Work out the finished part from the listing and answer in its coordinate system (mm). A direction names the side the tool comes from. Coordinates: 2 decimals unless noted, no trailing zeros. Order: outer loops, then holes, each group sorted by start corner. A loop starts at its lowest first (then second) coordinate and runs counter-clockwise, first axis right, second up. Notation, with made-up numbers: (21.25, 62.25) -> (58.25, 62.25) arc R10 ccw to (58.25, 75.25) -> close; hole circle Ø8 at (51, 85). An arc over 180 degrees is marked (long way). Use one line per item in the form item = value.
Autodesk Inventor part; units mm, degrees
ref_plane "type_gl_n_bm_XY" through (0, 0, 0) normal (1, 0, 0) x (0, -1, 0)
ref_plane "type_gl_n_bm_YZ" through (0, 0, 0) normal (0, -1, 0) x (0, 0, -1)
ref_plane "type_gl_n_bm_ZX" through (0, 0, 0) normal (0, 0, -1) x (1, 0, 0)
sketch "Sketch_1" plane through (0, 0, 0) normal (1, 0, 0) x (0, 1, 0)
  line L0 (27.33, 32.99) -> (-27.33, 32.99)
  line L1 (-27.33, 32.99) -> (-32.99, 27.33)
  line L2 (-32.99, 27.33) -> (-32.99, -27.33)
  line L3 (-32.99, -27.33) -> (-27.33, -32.99)
  line L4 (-27.33, -32.99) -> (27.33, -32.99)
  line L5 (27.33, -32.99) -> (32.99, -27.33)
  line L6 (32.99, -27.33) -> (32.99, 27.33)
  line L7 (32.99, 27.33) -> (27.33, 32.99)
extrude "Extrusion1" add sketch "Sketch_1" along normal blind 8
sketch "Sketch_2" plane through (0, 0, 0) normal (0, 0, 1) x (1, 0, 0)
  line L0 (40, 0) -> (8, 0)
  line L1 (8, 0) -> (8, 30)
  line L2 (8, 30) -> (40, 30)
  line L3 (40, 30) -> (40, 0)
  line L4 (40, 0) -> (8, 0)
revolve "Revolution1" add sketch "Sketch_2" angle 360 about axis through (40, 0, 0) along (1, 0, 0)
sketch "Sketch_3" plane through (40, 0, 0) normal (1, 0, 0) x (0, 0, -1)
  line L0 (-33, 27.34) -> (-33, -27.34)
  line L1 (-33, -27.34) -> (-27.34, -33)
  line L2 (-27.34, -33) -> (27.34, -33)
  line L3 (27.34, -33) -> (33, -27.34)
  line L4 (33, -27.34) -> (33, 27.34)
  line L5 (33, 27.34) -> (27.34, 33)
  line L6 (27.34, 33) -> (-27.34, 33)
  line L7 (-27.34, 33) -> (-33, 27.34)
extrude "Extrusion2" add sketch "Sketch_3" along normal blind 8
sketch "Sketch4" plane through (48, 0, 0) normal (1, 0, 0) x (0, 0, -1)
  point P0 (0, 0)
hole "Drilling 1" at (48, 0, 0) direction (-1, 0, 0) diameter 38.15 depth 8
sketch "Sketch5" plane through (40, 0, 0) normal (1, 0, 0) x (0, 0, -1)
  point P0 (0, 0)
hole "Drilling 2" at (40, 0, 0) direction (-1, 0, 0) diameter 50 depth 40
sketch "Sketch_7" plane through (0, 26.87, 0) normal (0, 1, 0) x (1, 0, 0)
  line L0 (13, 26.87) -> (8, 26.87)
  line L1 (8, 26.87) -> (8, 31.12)
  line L2 (8, 31.12) -> (13, 31.12)
  line L3 (13, 31.12) -> (13, 26.87)
  line L4 (13, 26.87) -> (8, 26.87)
revolve "Revolution2" add sketch "Sketch_7" angle 360 about axis through (13, 26.87, -26.87) along (1, 0, 0)
sketch "Sketch_8" plane through (0, 26.87, 0) normal (0, 1, 0) x (1, 0, 0)
  line L0 (13, -26.87) -> (8, -26.87)
  line L1 (8, -26.87) -> (8, -22.62)
  line L2 (8, -22.62) -> (13, -22.62)
  line L3 (13, -22.62) -> (13, -26.87)
  line L4 (13, -26.87) -> (8, -26.87)
revolve "Revolution3" add sketch "Sketch_8" angle 360 about axis through (13, 26.87, 26.87) along (1, 0, 0)
sketch "Sketch8" plane through (48, 0, 0) normal (1, 0, 0) x (0, 0, -1)
  point P0 (-23.57, 23.57)
hole "Drilling 3" at (48, 23.57, 23.57) direction (-1, 0, 0) diameter 3.242 depth 8 countersink diameter 4 countersink angle 90
sketch "Sketch9" plane through (48, 0, 0) normal (1, 0, 0) x (0, 0, -1)
  point P0 (-23.57, -23.57)
hole "Drilling 4" at (48, -23.57, 23.57) direction (-1, 0, 0) diameter 3.242 depth 8 countersink diameter 4 countersink angle 90
sketch "Sketch10" plane through (48, 0, 0) normal (1, 0, 0) x (0, 0, -1)
  point P0 (23.57, 23.57)
hole "Drilling 5" at (48, 23.57, -23.57) direction (-1, 0, 0) diameter 3.242 depth 8 countersink diameter 4 countersink angle 90
sketch "Sketch11" plane through (48, 0, 0) normal (1, 0, 0) x (0, 0, -1)
  point P0 (23.57, -23.57)
hole "Drilling 6" at (48, -23.57, -23.57) direction (-1, 0, 0) diameter 3.242 depth 8 countersink diameter 4 countersink angle 90
sketch "Sketch_9" plane through (0, -26.87, 0) normal (0, 1, 0) x (1, 0, 0)
  line L0 (13, 26.87) -> (8, 26.87)
  line L1 (8, 26.87) -> (8, 31.12)
  line L2 (8, 31.12) -> (13, 31.12)
  line L3 (13, 31.12) -> (13, 26.87)
  line L4 (13, 26.87) -> (8, 26.87)
revolve "Revolution4" add sketch "Sketch_9" angle 360 about axis through (13, -26.87, -26.87) along (1, 0, 0)
sketch "Sketch_10" plane through (0, -26.87, 0) normal (0, 1, 0) x (1, 0, 0)
  line L0 (13, -26.87) -> (8, -26.87)
  line L1 (8, -26.87) -> (8, -22.62)
  line L2 (8, -22.62) -> (13, -22.62)
  line L3 (13, -22.62) -> (13, -26.87)
  line L4 (13, -26.87) -> (8, -26.87)
revolve "Revolution5" add sketch "Sketch_10" angle 360 about axis through (13, -26.87, 26.87) along (1, 0, 0)
sketch "Sketch_33" plane through (0, 0, 0) normal (0, 1, 0) x (-1, 0, 0)
  line L0 (0, -17.5) -> (0, 17.5)
  line L1 (0, 17.5) -> (-33, 17.5)
  arc A0 (-33, 17.5) -> (-38, 12.5) centre (-33, 12.5) ccw
  line L2 (-38, 12.5) -> (-38, -12.5)
  arc A1 (-38, -12.5) -> (-33, -17.5) centre (-33, -12.5) ccw
  line L3 (-33, -17.5) -> (0, -17.5)
extrude "Extrusion3" cut sketch "Sketch_33" along normal blind 33
ref_plane "type_gl_n_bm_XY" through (0, 0, 0) normal (1, 0, 0) x (0, -1, 0)
ref_plane "type_gl_n_bm_YZ" through (0, 0, 0) normal (0, -1, 0) x (0, 0, -1)
ref_plane "type_gl_n_bm_ZX" through (0, 0, 0) normal (0, 0, -1) x (1, 0, 0)
properties part number "GL20NU1 Y Motor bracket"
(1) Each of these flat-tipped pins is pushed along its axis until it touches: P1, Ø3, axis at x = 26, y = -7.5, coming from the -Z side; P2, Ø5, axis at x = 21.5, y = 15.5, coming from the -Z side; P3, Ø8, axis at x = 26, z = -7.5, coming from the +Y side; P4, Ø3, axis at y = -9.5, z = 15, coming from the +X side. Where does it stop, or does it pass through?
Data:
P1 = -29.39
P2 = -27.04
P3 = -22.2
P4 = 48
(2) Straight lines are drawn through the part: line 1 along Z through (x, y) = (43.25, -23.57); line 2 along Y through (x, z) = (42, -23). For each, find the intervals that lie inside material, in ascending order.
Data:
line_1 = -33 to -25.19, -21.95 to 21.95, 25.19 to 33
line_2 = -33 to -25.09, -22.05 to 22.05, 25.09 to 33
(3) Section C-C on x = 6 is taken. Write down the section's boundary in (y, z).
Data:
outline = (-32.99, -27.33) -> (-27.33, -32.99) -> (27.33, -32.99) -> (32.99, -27.33) -> (32.99, -17.5) -> (17.85, -17.5) arc R25 cw (long way) to (17.85, 17.5) -> (32.99, 17.5) -> (32.99, 27.33) -> (27.33, 32.99) -> (-27.33, 32.99) -> (-32.99, 27.33) -> close
(4) Section A-A on z = 0 is taken. Write down the section's boundary in (x, y) (3 decimals).
Data:
outline = (0, -32.99) -> (8, -32.99) -> (8, -30) -> (40, -30) -> (40, -33) -> (48, -33) -> (48, -19.075) -> (40, -19.075) -> (40, -25) -> (0, -25) -> close; (38, 25) -> (40, 25) -> (40, 19.075) -> (48, 19.075) -> (48, 33) -> (40, 33) -> (40, 30) -> (38, 30) -> close
(5) Section D-D on z = 14.5 is taken. Write down the section's boundary in (x, y).
Data:
outline = (0, -32.99) -> (8, -32.99) -> (8, -26.26) -> (40, -26.26) -> (40, -33) -> (48, -33) -> (48, -12.39) -> (40, -12.39) -> (40, -20.37) -> (0, -20.37) -> close; (37.58, 20.37) -> (40, 20.37) -> (40, 12.39) -> (48, 12.39) -> (48, 33) -> (40, 33) -> (40, 26.26) -> (37.58, 26.26) -> close
(6) Section B-B on y = 0 is taken. Write down the section's boundary in (x, z) (3 decimals), plus the area to 3 significant figures.
Data:
outline = (0, -32.99) -> (8, -32.99) -> (8, -30) -> (40, -30) -> (40, -33) -> (48, -33) -> (48, -19.075) -> (40, -19.075) -> (40, -25) -> (0, -25) -> close; (0, 25) -> (40, 25) -> (40, 19.075) -> (48, 19.075) -> (48, 33) -> (40, 33) -> (40, 30) -> (8, 30) -> (8, 32.99) -> (0, 32.99) -> close
area = 671 mm²
(7) Which of the six approach directions +Z, -Z, +X, -X, +Y, -Y give full straight-line access (tool end or side, diameter ignored) to faces 5 (the flat face through (40, 25, 17)), 6 (the cylindrical face through (36.5, 22.5, -16.07)), 7 (the cylindrical face through (43.757, 21.963, 23.781))?
Data:
face_5 = none
face_6 = -X, +Y
face_7 = +X
(8) The mould has two halves that part along Y. Classify faces 1 (the cylindrical face through (43.76, -23.64, 25.19)), 2 (the cylindrical face through (43.944, -18.913, 2.483)), 3 (the flat face through (43.94, -30.21, -30.13)), 4 (the flat face through (4, 32.99, 22)): released by +Y, released by -Y, zero draft, split by the parting line, or undercut.
Data:
face_1 = undercut
face_2 = undercut
face_3 = released by -Y
face_4 = released by +Y
